Model file for the job. Use its own axes, mm. Face numbers are marked on the shaded views. A direction names the side the tool comes from. Coordinates: 2 decimals unless noted, no trailing zeros. Write each loop counter-clockwise with the first axis right and the second up, starting at its lowest first coordinate (ties: lowest second). Pieces come first, ordered by that corner, then holes. Notation, with made-up numbers: (34.25, -28.75) - (89.25, -28.75) arc R30 ccw to (89.25, 10.25) - close; hole circle Ø2 at (20.5, 66.5). An arc over 180 degrees is marked (long way). Put each result on its own line as item: value. Start each with the question number.
1. Saw through at C-C, the plane y = 7.25. Write the cut outline in (x, z).
2. Saw through at B-B, the plane x = 16.5. Write the cut outline in (y, z).
3. Drill centre lines: L1, parallel to Z at x = 34, y = 12.75; L2, parallel to Y at x = 25.5, z = -16.75; L3, parallel to Y at x = 17, z = -1.5. Where is each one in solid material? Low to high. Write a range as from..to.
4. Saw through at D-D, the plane x = 47.5. Write the cut outline in (y, z), plus the area to 3 significant figures.
5. Saw through at A-A, the plane y = 1.5. Write the cut outline in (x, z).
6. Which spindle directions (+Z, -Z, +X, -X, +Y, -Y) get a long thin tool onto all of the face, cutting with end or side? Do the marked faces 1 and 2. Say none if no direction does.
7. Pull direction Z, two halves, no side cores. Call the marked faces 3, 4 and 5: released by +Z, released by -Z, zero draft, split by the parting line, or undercut.
8. Drop flat-ended pins along their axis: P1, Ø4, axis at x = 31.5, z = -21, coming from the +Y side; P2, Ø9, axis at y = 7.5, z = -16, coming from the -X side. Give the stop position or say it passes through.
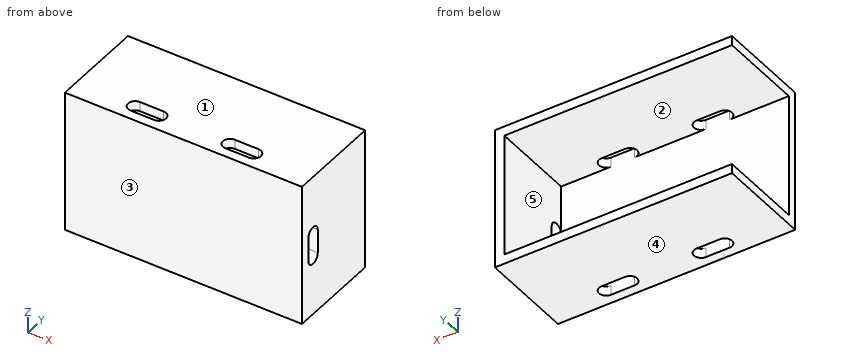
```python
from build123d import *

# Parameters (mm, degrees)
EXTRUDE_THIN1_DEPTH     = 18
SKETCH2_W               = 50
SKETCH2_H               = 30
BOSS_EXTRUDE1_DEPTH     = 2
CUT_EXTRUDE1_DEPTH      = 62.02458521
CUT_EXTRUDE1_DEPTH_BACK = 62.02458521
CUT_EXTRUDE2_DEPTH      = 60.39696962
CUT_EXTRUDE2_DEPTH_BACK = 60.39696962


with BuildPart() as part:
    # Sketch1 → Extrude-Thin1 (new body)
    with BuildSketch(Plane(origin=(0, 0, 0), x_dir=(1, 0, 0), z_dir=(0, 1, 0))):
        Polygon((0, 28), (48, 28), (48, 2), (0, 2), (0, 0), (50, 0), (50, 30), (0, 30), align=None)
    extrude(amount=EXTRUDE_THIN1_DEPTH)

    # Sketch2 → Boss-Extrude1 (add)
    with BuildSketch(Plane.XZ):
        with Locations((25, -15)):
            Rectangle(SKETCH2_W, SKETCH2_H)
    extrude(amount=BOSS_EXTRUDE1_DEPTH)

    # Sketch3 → Cut-Extrude1 (cut, two sides: drawn at the far end of the back side and taken through both)
    with BuildSketch(Plane.XY.offset(-CUT_EXTRUDE1_DEPTH_BACK)):
        with BuildLine():
            Line((12.5, 3), (17.5, 3))
            ThreePointArc((17.5, 3), (19, 1.5), (17.5, 0))
            Line((17.5, 0), (12.5, 0))
            ThreePointArc((12.5, 0), (11, 1.5), (12.5, 3))
        make_face()
        with BuildLine():
            Line((37.5, 3), (32.5, 3))
            ThreePointArc((32.5, 3), (31, 1.5), (32.5, 0))
            Line((32.5, 0), (37.5, 0))
            ThreePointArc((37.5, 0), (39, 1.5), (37.5, 3))
        make_face()
    extrude(amount=CUT_EXTRUDE1_DEPTH + CUT_EXTRUDE1_DEPTH_BACK, mode=Mode.SUBTRACT)

    # Sketch4 → Cut-Extrude2 (cut, two sides: drawn at the far end of the back side and taken through both)
    with BuildSketch(Plane.ZY.offset(-48).offset(-CUT_EXTRUDE2_DEPTH_BACK)):
        with BuildLine():
            Line((-17.5, 3), (-12.5, 3))
            ThreePointArc((-12.5, 3), (-11, 1.5), (-12.5, 0))
            Line((-12.5, 0), (-17.5, 0))
            ThreePointArc((-17.5, 0), (-19, 1.5), (-17.5, 3))
        make_face()
    extrude(amount=CUT_EXTRUDE2_DEPTH + CUT_EXTRUDE2_DEPTH_BACK, mode=Mode.SUBTRACT)


solid = part.part
```
Final values:
1. outline: (0, -30) - (50, -30) - (50, 0) - (0, 0) - (0, -2) - (48, -2) - (48, -28) - (0, -28) - close
2. outline: (-2, -30) - (0, -30) - (0, 0) - (-2, 0) - close; (3, -30) - (18, -30) - (18, -28) - (3, -28) - close; (3, -2) - (18, -2) - (18, 0) - (3, 0) - close
3. L1: z = -30..-28, -2..0
3. L2: y = -2..0
3. L3: y = -2..0, 3..18
4. outline: (-2, -30) - (18, -30) - (18, -28) - (0, -28) - (0, -2) - (18, -2) - (18, 0) - (-2, 0) - close
4. area: 132 mm²
5. outline: (0, -30) - (11, -30) - (11, -28) - (0, -28) - close; (0, -2) - (11, -2) - (11, 0) - (0, 0) - close; (19, -30) - (31, -30) - (31, -28) - (19, -28) - close; (19, -2) - (31, -2) - (31, 0) - (19, 0) - close; (39, -30) - (50, -30) - (50, -19) - (48, -19) - (48, -28) - (39, -28) - close; (39, -2) - (48, -2) - (48, -11) - (50, -11) - (50, 0) - (39, 0) - close
6. face 1: +Z, +X, -X, +Y, -Y
6. face 2: -X, +Y
7. face 3: zero draft
7. face 4: released by -Z
7. face 5: undercut
8. P1: stops at y = 0
8. P2: stops at x = 48
